```python
from build123d import *

# Parameters (mm, degrees)
F0_W     = 2000
F0_H     = 750
F1_DEPTH = 50
F2_T     = -18
F3_DEPTH = 25
F5_DEPTH = 46.5
F6_W     = 1964
F6_H     = 714
F7_DEPTH = 3.5


with BuildPart() as f1:
    # F0 (on Top) → F1 (new body)
    with BuildSketch(Plane.XY):
        Rectangle(F0_W, F0_H)
    extrude(amount=F1_DEPTH)

    # F2
    f2_openings = [f1.faces().sort_by_distance(p)[0] for p in [
        (0, 0, 50),
    ]]
    offset(amount=F2_T, openings=f2_openings)

    # F3 (cut): a face of the model
    f3_faces = [f1.faces().sort_by_distance(p)[0] for p in [
        (0, 0, 18),
    ]]
    extrude(f3_faces, amount=-F3_DEPTH, mode=Mode.SUBTRACT)

    # F4 (on face) → F5 (join)
    with BuildSketch(Plane.XY):
        Polygon((9, 357), (0, 357), (-9, 357), (-18, -357), (0, -357), align=None)
    extrude(amount=F5_DEPTH)

    # F6 (on face) → F7 (cut)
    with BuildSketch(Plane.XY.offset(50)):
        Polygon((982, 362), (-982, 362), (-987, 362), (-987, 357), (-987, -357), (-987, -362), (-982, -362), (982, -362), (987, -362), (987, -357), (987, 357), (987, 362), align=None)
        Rectangle(F6_W, F6_H, mode=Mode.SUBTRACT)
    extrude(amount=-F7_DEPTH, mode=Mode.SUBTRACT)


solid = f1.part
```
The listing builds one solid part. Answer for the finished solid, in the listing's coordinates (mm). A direction names the side the tool comes from. Coordinates: 2 decimals unless noted, no trailing zeros. Write each loop counter-clockwise with the first axis right and the second up, starting at its lowest first coordinate (ties: lowest second). Pieces come first, ordered by that corner, then holes. Notation, with made-up numbers: (45.25, 25.5) - (101.25, 25.5) arc R27 cw to (101.25, 53.5) - close; hole circle Ø7 at (-5, 74.5). An arc over 180 degrees is marked (long way). Return JSON: item names as keys, results as strings. Group by question number.
1. A cutting plane is placed at C-C, the plane y = 68. Determine the outline of the cut face in (x, z).
2. Which of the six approach directions +Z, -Z, +X, -X, +Y, -Y give full straight-line access (tool end or side, diameter ignored) to faces 1 (the flat face through (-5, 363, 50)), 2 (the flat face through (-5, 2, 46.5)), 3 (the flat face through (484, -357, 24))?
3. A cutting plane is placed at A-A, the plane x = -333.5. Determine the outline of the cut face in (y, z).
4. Straight lines are drawn through the part: L1, parallel to Y at x = 120, z = 37.5; L2, parallel to X at y = -180.5, z = 15; L3, parallel to X at y = 99.5, z = 13.5. For each, find the intervals that lie inside material, in ascending order.
5. A cutting plane is placed at B-B, the plane z = 22. Determine the outline of the cut face in (x, y).
6. Determine the mould class of faces 4 (the flat face through (-14, 375, 25)), 5 (the flat face through (489, 357, 24)), 6 (the flat face through (1000, -5, 25)) for opening direction X: released by +X, released by -X, zero draft, split by the parting line, or undercut.
Ans:
{
 "1": {"outline": "(-1000, 0) - (-982, 0) - (-982, 46.5) - (-987, 46.5) - (-987, 50) - (-1000, 50) - close; (-12.64, 0) - (5.36, 0) - (5.36, 46.5) - (-12.64, 46.5) - close; (982, 0) - (1000, 0) - (1000, 50) - (987, 50) - (987, 46.5) - (982, 46.5) - close"},
 "2": {"face 1": "+Z, +X, -X, +Y, -Y", "face 2": "+Z", "face 3": "+Z, -Z"},
 "3": {"outline": "(-375, 0) - (-357, 0) - (-357, 46.5) - (-362, 46.5) - (-362, 50) - (-375, 50) - close; (357, 0) - (375, 0) - (375, 50) - (362, 50) - (362, 46.5) - (357, 46.5) - close"},
 "4": {"L1": "-375 to -357, 357 to 375", "L2": "-1000 to -982, -15.78 to 2.22, 982 to 1000", "L3": "-1000 to -982, -12.25 to 5.75, 982 to 1000"},
 "5": {"outline": "(-1000, -375) - (1000, -375) - (1000, 375) - (-1000, 375) - close; hole (-982, -357) - (-18, -357) - (-9, 357) - (-982, 357) - close; hole (0, -357) - (982, -357) - (982, 357) - (9, 357) - close"},
 "6": {"face 4": "zero draft", "face 5": "undercut", "face 6": "released by +X"}
}
